Model file for the job. Use its own axes, mm. Round coordinates to 2 decimals unless told otherwise and drop trailing zeros. Loops run counter-clockwise (first coordinate to the right, second up) from the corner with the lowest first, then second, coordinate; pieces in that order, holes last. Notation, with made-up numbers: (-5.75, 41) - (5.25, 41) arc R23 ccw to (5.25, 63) - close; hole circle Ø7 at (14.5, -31.75). An arc over 180 degrees is marked (long way). Use one line per item in the form item = value.
from build123d import *

# Parameters (mm, degrees)
PAD015_DEPTH                        = 3
SKETCH054_R                         = 1.65
POCKET018_DEPTH                     = 358.938883
POCKET018_DEPTH_BACK                = 361.938883
BODY001003005003004_PLACEMENT_ANGLE = 60
CLONE004_PLACEMENT_ANGLE            = 142


with BuildPart() as part:
    # Sketch053 → Pad015 (new body)
    with BuildSketch(Plane.XY):
        with BuildLine():
            ThreePointArc((152.005097, 113.785532), (84.992984, 169.790723), (0, 189.875477))
            Line((0, 189.875477), (0, 196.875477))
            ThreePointArc((157.608957, 117.98038), (88.126358, 176.050273), (0, 196.875477))
            ThreePointArc((152.005097, 113.785532), (156.904451, 113.081026), (157.608957, 117.98038))
        make_face()
    pad015 = extrude(amount=PAD015_DEPTH)

    # Sketch054 → Pocket018 (cut, two sides)
    with BuildSketch(Plane.XY) as pocket018_sk:
        with Locations((150.82443, 121.020933)):
            Circle(SKETCH054_R)
        with BuildLine():
            ThreePointArc((0, 191.725477), (1.65, 193.375477), (0, 195.025477))
            Line((0, 191.725477), (0, 195.025477))
        make_face()
    pocket018 = extrude(amount=-POCKET018_DEPTH, mode=Mode.SUBTRACT) + extrude(pocket018_sk.sketch, amount=POCKET018_DEPTH_BACK, mode=Mode.SUBTRACT)

    # Mirrored020: Pad015, Pocket018 across Sketch053 V_Axis
    add(pad015.mirror(Plane(origin=(0, 0, 0), x_dir=(0, 0, 1), z_dir=(1, 0, 0))))
    add(pocket018.mirror(Plane(origin=(0, 0, 0), x_dir=(0, 0, 1), z_dir=(1, 0, 0))), mode=Mode.SUBTRACT)


with BuildPart() as part_1:
    # Body001003005003004 placement: moved
    add(part.part.rotate(Axis((0, 0, 0), (0, 0, 1)), BODY001003005003004_PLACEMENT_ANGLE))


with BuildPart() as part_2:
    # Clone004 placement: moved
    add(part_1.part.moved(Location((1306, 669, 0))).rotate(Axis((1306, 669, 0), (0, 0, 1)), CLONE004_PLACEMENT_ANGLE))


solid = part_2.part
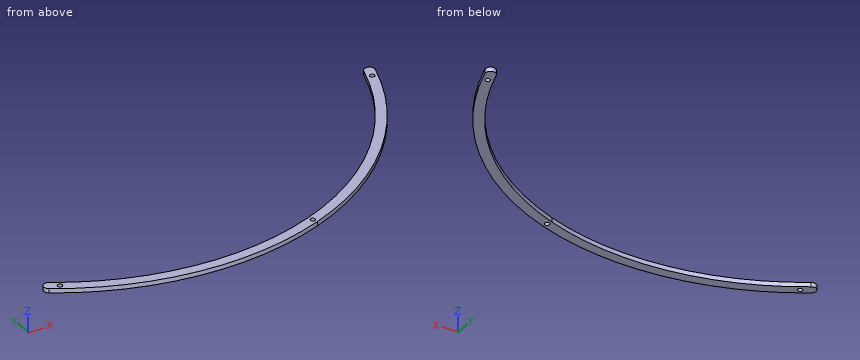
1. Cut at A-A, the plane z = 2.05. Give the cut face in (x, y), plus the area to 3 significant figures.
Geometry check:
outline = (1204.06, 500.57) arc R196.88 ccw to (1379.75, 486.46) arc R196.88 ccw to (1496.33, 618.65) arc R3.5 ccw to (1489.56, 620.44) arc R189.88 cw to (1377.13, 492.95) arc R189.88 cw to (1207.69, 506.56) arc R3.5 ccw to start; hole circle Ø3.3 at (1211.49, 500.29); hole circle Ø3.3 at (1378.44, 489.71); hole circle Ø3.3 at (1491.18, 613.29)
area = 2,530 mm^2
2. Cut at B-B, the plane y = 557. Give the cut face in (x, z), plus the area to 3 significant figures.
Geometry check:
outline = (1459.33, 0) - (1467.91, 0) - (1467.91, 3) - (1459.33, 3) - close
area = 25.8 mm^2
3. Flat gauge pins, fed straight in: pin 1 (1.5 mm diameter, centred on x = 1253, z = 2, fed in from +Y); pin 2 (3 mm diameter, centred on x = 1211.49, y = 500.29, fed in from +Z); pin 3 (5.5 mm diameter, centred on x = 1378.44, y = 489.71, fed in from -Z). Where does each tip first touch, or does it go through?
Geometry check:
pin_1 = 486.89
pin_2 = through
pin_3 = 0
4. Wall check: probe 1 along Y at (x, z) = (1302, 1); probe 2 along Y at (x, z) = (1321, 0.3); probe 3 along X at (y, z) = (495, 1.95). Give the ranges that are in metal, low to high.
Geometry check:
probe_1 = 472.17 to 479.17
probe_2 = 472.7 to 479.72
probe_3 = 1213.89 to 1230, 1382 to 1398.11
5. Cut at C-C, the plane x = 1406. Give the cut face in (y, z).
Geometry check:
outline = (499.41, 0) - (507.59, 0) - (507.59, 3) - (499.41, 3) - close
